Could you check a few things on this model? Use its own coordinates, in mm. Face numbers are marked on the shaded views. A direction names the side the tool comes from. Coordinates: 2 decimals unless noted, no trailing zeros. Loops run counter-clockwise (first coordinate to the right, second up) from the corner with the lowest first, then second, coordinate; pieces in that order, holes last.
from build123d import *

# Parameters (mm, degrees)
ESQUISSE2_R        = 1.5
BOSS_EXTRU_2_DEPTH = 3


with BuildPart() as part:
    # Esquisse2 → Boss.-Extru.2 (new body)
    with BuildSketch(Plane.XY):
        with BuildLine():
            Line((4.526650681, 18.4), (18.526650681, 18.4))
            ThreePointArc((18.526650681, 18.4), (31.026650681, 5.9), (18.526650681, -6.6))
            Line((18.526650681, -6.6), (4.526650681, -6.6))
            ThreePointArc((4.526650681, -6.6), (-7.973349319, 5.9), (4.526650681, 18.4))
        make_face()
        with Locations((11.526650681, 15.4)):
            Circle(ESQUISSE2_R, mode=Mode.SUBTRACT)
        with Locations((11.526650681, -3.6)):
            Circle(ESQUISSE2_R, mode=Mode.SUBTRACT)
        Polygon((0, 0), (0, 11.8), (23, 11.8), (23, 8.4), (24.940257674, 8.4), (24.940257674, 3.4), (23, 3.4), (23, 0), align=None, mode=Mode.SUBTRACT)
    extrude(amount=BOSS_EXTRU_2_DEPTH)


solid = part.part
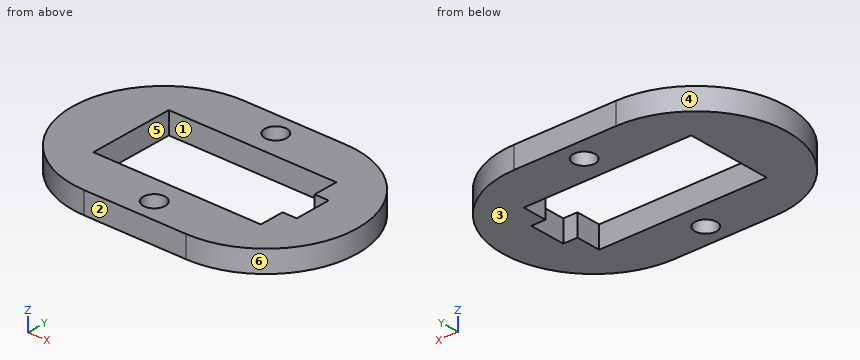
(1) Imagine slicing it at C-C, the plane z = 0.5. Write out the boundary of the cut face in (x, y), and give its area (3 significant figures).
Answers:
outline: (4.53, -6.6) - (18.53, -6.6) arc R12.5 ccw to (18.53, 18.4) - (4.53, 18.4) arc R12.5 ccw to start; hole (0, 0) - (23, 0) - (23, 3.4) - (24.94, 3.4) - (24.94, 8.4) - (23, 8.4) - (23, 11.8) - (0, 11.8) - close; hole circle Ø3 at (11.53, -3.6); hole circle Ø3 at (11.53, 15.4)
area: 546 mm2
(2) For pin 1 (4 mm diameter, centred on x = 11.53, y = -3.6, fed in from -Z); pin 2 (0.9 mm diameter, centred on y = 10, z = 1.5, fed in from -X); pin 3 (1 mm diameter, centred on x = 23.5, z = 2, fed in from +Y); pin 4 (0.9 mm diameter, centred on y = 1.5, z = 1.5, fed in from -X), each with a flat end and sliding along its axis, tell me the tip position at first contact or that it passes through.
Answers:
pin 1: stops at z = 0
pin 2: stops at x = -7.43
pin 3: stops at y = 17.57
pin 4: stops at x = -7.33
(3) Imagine slicing it at B-B, the plane y = 5.9. Write out the boundary of the cut face in (x, z), and give its area (3 significant figures).
Answers:
outline: (-7.97, 0) - (0, 0) - (0, 3) - (-7.97, 3) - close; (24.94, 0) - (31.03, 0) - (31.03, 3) - (24.94, 3) - close
area: 42.2 mm2
(4) Imagine slicing it at D-D, the plane x = -4.5. Write out the boundary of the cut face in (y, z), and give its area (3 significant figures).
Answers:
outline: (-2.75, 0) - (14.55, 0) - (14.55, 3) - (-2.75, 3) - close
area: 51.9 mm2
(5) I need wall thicknesses on probe 1 along Y at (x, z) = (19, 2.1); probe 2 along X at (y, z) = (5.75, 1.45); probe 3 along X at (y, z) = (7.25, 1.15). Which ranges of each line are inside material? Lowest first, please.
Answers:
probe 1: y = -6.59 to 0, 11.8 to 18.39
probe 2: x = -7.97 to 0, 24.94 to 31.03
probe 3: x = -7.9 to 0, 24.94 to 30.95
(6) We'd pull the mould along X, two halves only. Please class the marked faces 3, 4, 5 and 6: +X half, -X half, draft (parallel to the pull), parting line (faces both ways), or undercut.
Answers:
face 3: draft
face 4: -X half
face 5: undercut
face 6: +X half
(7) Which directions (+Z, -Z, +X, -X, +Y, -Y) give clear straight access to the entire face, cutting with the end or side of a thin tool? Please do the marked faces 1 and 2.
Answers:
face 1: +Z, -Z
face 2: +Z, -Z, +X, -X, -Y
(8) Imagine slicing it at A-A, the plane x = 5. Write out the boundary of the cut face in (y, z).
Answers:
outline: (-6.6, 0) - (0, 0) - (0, 3) - (-6.6, 3) - close; (11.8, 0) - (18.4, 0) - (18.4, 3) - (11.8, 3) - close
